Check sheet for the modelled part. Datum: model origin and axes. Units: mm. Face numbers are marked on the shaded views. A direction names the side the tool comes from. Give positions to 0.01 mm unless a question says otherwise; leave off trailing zeros. Write each loop counter-clockwise with the first axis right and the second up, starting at its lowest first coordinate (ties: lowest second). Pieces come first, ordered by that corner, then holes.
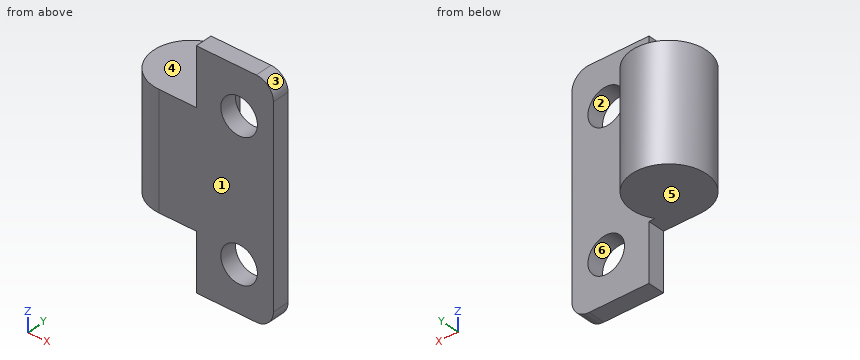
from build123d import *

# Parameters (mm, degrees)
EXTRUDE_1_DEPTH          = 10
CUT_EXTRUDE_1_DEPTH      = 16.006678513
CUT_EXTRUDE_1_DEPTH_BACK = 16.006678513
SKETCH_2_R               = 1.6
SKETCH_2_W               = 6.52
SKETCH_2_H               = 5
FILLET_1_R               = 1.5


with BuildPart() as part:
    # 草图1 → 凸台-拉伸1 (new, symmetric)
    with BuildSketch(Plane.XY):
        with BuildLine():
            Line((0, -3.26), (10, -3.26))
            Line((10, -3.26), (10, -1.76))
            Line((10, -1.76), (2.744084547, -1.76))
            ThreePointArc((2.744084547, -1.76), (-1.563649577, 2.860524427), (0, -3.26))
        make_face()
    extrude(amount=EXTRUDE_1_DEPTH, both=True)

    # 草图2 → 切除-拉伸1 (cut, two sides: drawn at the far end of the back side and taken through both)
    with BuildSketch(Plane(origin=(0, -1.76, 0), x_dir=(1, 0, 0), z_dir=(0, 1, 0)).offset(-CUT_EXTRUDE_1_DEPTH_BACK)):
        with Locations(Location((7, 6, 0), (0, 0, 180))):
            Circle(SKETCH_2_R)
        with Locations((7, -6)):
            Circle(SKETCH_2_R)
        with Locations((0, 7.5)):
            Rectangle(SKETCH_2_W, SKETCH_2_H)
        with Locations((0, -7.5)):
            Rectangle(SKETCH_2_W, SKETCH_2_H)
    extrude(amount=CUT_EXTRUDE_1_DEPTH + CUT_EXTRUDE_1_DEPTH_BACK, mode=Mode.SUBTRACT)

    # 圆角1
    fillet_1_edges = [part.edges().sort_by_distance(p)[0] for p in [
        (10, -2.51, 10),
        (10, -2.51, -10),
    ]]
    fillet(fillet_1_edges, radius=FILLET_1_R)


solid = part.part
1) Sectioned sample at C-C on y = 0. Record the boundary of the cut face in (x, z), then the cut area to 3 significant figures.
2) Gauge pin test, flat ends, axial feed: pin 1 (2 mm diameter, centred on x = -0.5, y = -1, fed in from -Z); pin 2 (5 mm diameter, centred on x = 7, z = -6, fed in from +Y); pin 3 (1.5 mm diameter, centred on x = 6.5, y = -0.5, fed in from -Z); pin 4 (2 mm diameter, centred on x = -1.5, y = 1.5, fed in from +Z). Record the tip position at first contact, or that the pin passes through.
3) Sectioned sample at A-A on x = 7. Record the boundary of the cut face in (y, z), then the cut area to 3 significant figures.
4) Access from +Z, -Z, +X, -X, +Y, -Y to the whole of each face (thin tool, end or side, straight path). Record for the marked faces 4, 5 and 6.
5) Draft check along Z on the marked faces 1, 2 and 3. Enter one of: +Z half, -Z half, draft (parallel to the pull), parting line (faces both ways), or undercut.
6) Scan lines: L1, parallel to Z at x = 7, y = -2.35; L2, parallel to X at y = -2.6, z = -6; L3, parallel to Y at x = 5.75, z = -0.5. Record each from-to range of solid material in increasing order.
7) Sectioned sample at B-B on z = -3.25. Record the boundary of the cut face in (x, y).
Answers below:
1. outline: (-3.26, -5) - (3.26, -5) - (3.26, 5) - (-3.26, 5) - close
1. area: 65.2 mm2
2. pin 1: stops at z = -5
2. pin 2: stops at y = -1.76
2. pin 3: passes through
2. pin 4: stops at z = 5
3. outline: (-3.26, -10) - (-1.76, -10) - (-1.76, -7.6) - (-3.26, -7.6) - close; (-3.26, -4.4) - (-1.76, -4.4) - (-1.76, 4.4) - (-3.26, 4.4) - close; (-3.26, 7.6) - (-1.76, 7.6) - (-1.76, 10) - (-3.26, 10) - close
3. area: 20.4 mm2
4. face 4: +Z, -X, +Y, -Y
4. face 5: -Z, -X, +Y, -Y
4. face 6: +Y, -Y
5. face 1: draft
5. face 2: undercut
5. face 3: +Z half
6. L1: z = -10 to -7.6, -4.4 to 4.4, 7.6 to 10
6. L2: x = 3.26 to 5.4, 8.6 to 10
6. L3: y = -3.26 to -1.76
7. outline: (0, -3.26) - (10, -3.26) - (10, -1.76) - (2.74, -1.76) arc R3.26 ccw (long way) to start
